from build123d import *

# Parameters (mm, degrees)
SKETCH1_W           = 8.25
SKETCH1_H           = 32.8
SKETCH2_R           = 5.6
CUT_EXTRUDE1_DEPTH  = 0.75
CUT_EXTRUDE2_START  = -0.1
SKETCH3_R           = 5.6
CUT_EXTRUDE2_DEPTH  = 0.1
CUT_EXTRUDE3_DEPTH  = 0.75
SKETCH5_R           = 3.2
BOSS_EXTRUDE3_DEPTH = 2.15
FILLET1_R           = 0.5
SKETCH6_R           = 6.1
SKETCH6_R_2         = 5.6
CUT_EXTRUDE4_DEPTH  = 0.65
FILLET2_R           = 0.5


with BuildPart() as part:
    # Sketch1 → Base-Revolve (revolve)
    with BuildSketch(Plane.XY, mode=Mode.PRIVATE) as base_revolve_sk:
        with Locations((4.125, 0)):
            Rectangle(SKETCH1_W, SKETCH1_H)
    revolve(base_revolve_sk.sketch.rotate(Axis((0, -16.4, 0), (0, 1, 0)), 90), axis=Axis((0, -16.4, 0), (0, 1, 0)))

    # Sketch2 → Cut-Extrude1 (cut)
    with BuildSketch(Plane.XZ.offset(16.4)):
        with Locations(Location((0, 0, 0), (0, 0, 270))):
            Circle(SKETCH2_R)
    extrude(amount=-CUT_EXTRUDE1_DEPTH, mode=Mode.SUBTRACT)

    # Sketch3 → Cut-Extrude2 (cut)
    with BuildSketch(Plane(origin=(0, 16.4, 0), x_dir=(-1, 0, 0), z_dir=(0, 1, 0)).offset(CUT_EXTRUDE2_START)):
        with Locations(Location((0, 0, 0), (0, 0, 270))):
            Circle(SKETCH3_R)
    extrude(amount=CUT_EXTRUDE2_DEPTH, mode=Mode.SUBTRACT)

    # Sketch4 → Cut-Extrude3 (cut)
    with BuildSketch(Plane(origin=(0, 16.3, 0), x_dir=(-1, 0, 0), z_dir=(0, 1, 0))):
        Polygon((3.225, -2.343099653), (3.225, 2.343099653), (-1.231840386, 3.791214877), (-3.986319227, 0), (-1.231840386, -3.791214877), align=None)
    extrude(amount=-CUT_EXTRUDE3_DEPTH, mode=Mode.SUBTRACT)

    # Sketch5 → Boss-Extrude3 (add)
    with BuildSketch(Plane(origin=(0, 15.55, 0), x_dir=(-1, 0, 0), z_dir=(0, 1, 0))):
        with Locations(Location((0, 0, 0), (0, 0, 270))):
            Circle(SKETCH5_R)
    extrude(amount=BOSS_EXTRUDE3_DEPTH)

    # Fillet1
    fillet1_edges = [part.edges().sort_by_distance(p)[0] for p in [
        (0, 17.7, 3.2),
    ]]
    fillet(fillet1_edges, radius=FILLET1_R)

    # Sketch6 → Cut-Extrude4 (cut)
    with BuildSketch(Plane.XZ.offset(16.3)):
        with Locations(Location((0, 0, 0), (0, 0, 270))):
            Circle(SKETCH6_R)
        with Locations(Location((0, 0, 0), (0, 0, 270))):
            Circle(SKETCH6_R_2, mode=Mode.SUBTRACT)
    extrude(amount=-CUT_EXTRUDE4_DEPTH, mode=Mode.SUBTRACT)

    # Fillet2
    fillet2_edges = [part.edges().sort_by_distance(p)[0] for p in [
        (0, -16.4, 8.25),
        (0, 16.4, 8.25),
    ]]
    fillet(fillet2_edges, radius=FILLET2_R)


solid = part.part
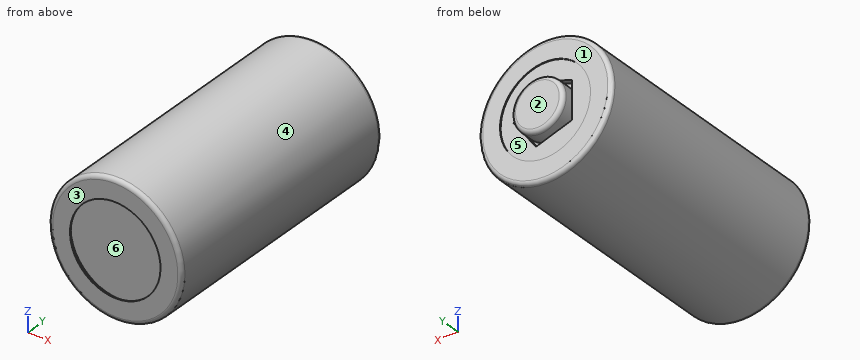
Model file for the job. Use its own axes, mm. Face numbers are marked on the shaded views. A direction names the side the tool comes from. Give positions to 0.01 mm unless a question says otherwise; leave off trailing zeros. Loops run counter-clockwise (first coordinate to the right, second up) from the corner with the lowest first, then second, coordinate; pieces in that order, holes last.
1) Saw through at B-B (y = 8.5). Write the cut outline in (x, z).
2) Tool access for the marked faces 1 and 2: list every direction of +Z, -Z, +X, -X, +Y, -Y with a clear straight run to the whole face (end or side of a thin tool).
3) Wall check: line 1 (Y direction, x = 3.25, z = 2.25); line 2 (Y direction, x = 5.25, z = -3.25); line 3 (X direction, y = 16.45, z = 0). Give the ranges that are in metal, low to high.
4) Flat gauge pins, fed straight in: pin 1 Ø2 at (y, z) = (-11.5, -1.5) entering from +X; pin 2 Ø1 at (x, z) = (1.5, 0) entering from -Y; pin 3 Ø2 at (x, y) = (1.5, -5) entering from -Z. Where does each tip first touch, or does it go through?
5) Pull direction Z, two halves, no side cores. Call the marked faces 3, 4, 5 and 6: +Z half, -Z half, draft (parallel to the pull), parting line (faces both ways), or undercut.
Answer block:
1. outline: circle Ø16.5 at (0, 0)
2. face 1: +Y
2. face 2: +Z, -Z, +X, -X, +Y
3. line 1: y = -15.65 to 16.3
3. line 2: y = -16.4 to 16.4
3. line 3: x = -3.2 to 3.2
4. pin 1: stops at x = 8.23
4. pin 2: stops at y = -15.65
4. pin 3: stops at z = -8.23
5. face 3: draft
5. face 4: parting line
5. face 5: undercut
5. face 6: undercut
